Could you check a few things on this drawing? It's one solid part, dimensions in mm from its lowest x, y, z. Round coordinates to 2 decimals unless told otherwise and drop trailing zeros. Write each loop counter-clockwise with the first axis right and the second up, starting at its lowest first coordinate (ties: lowest second). Pieces come first, ordered by that corner, then holes. Notation, with made-up numbers: (45.25, 83.25) -> (68.25, 83.25) arc R27 cw to (68.25, 116.25) -> close; hole circle Ø2 at (72, -22.5). An arc over 180 degrees is marked (long way). Put each result on its own line as item: value. Start each with the question number.
1) I want a section at C-C, the plane y = 7.5. List the corners of the cut face in (x, z) for me (1 decimal).
2) I want a section at B-B, the plane x = 325. List the corners of the cut face in (y, z) for me (1 decimal).
3) I want a section at D-D, the plane z = 105. List the corners of the cut face in (x, y) for me, then the cut area to 3 significant figures.
4) Will these pins go through, and if not, where does the flat tip stop? P1, Ø3, axis at y = 6.5, z = 207.5, coming from the +X side (1 decimal); P2, Ø4, axis at x = 204.5, y = 5.5, coming from the +Z side; P3, Ø3, axis at x = 330, y = 4.5, coming from the -Z side.
5) If I drill on line 1 along X through (y, z) = (8.25, 291) (1 decimal); line 2 along Z through (x, y) = (43, 6.5); line 3 along X through (y, z) = (6.5, 330.5) (1 decimal), over which ranges is the centre line in solid material (lowest first)? Write a range as [from, to].
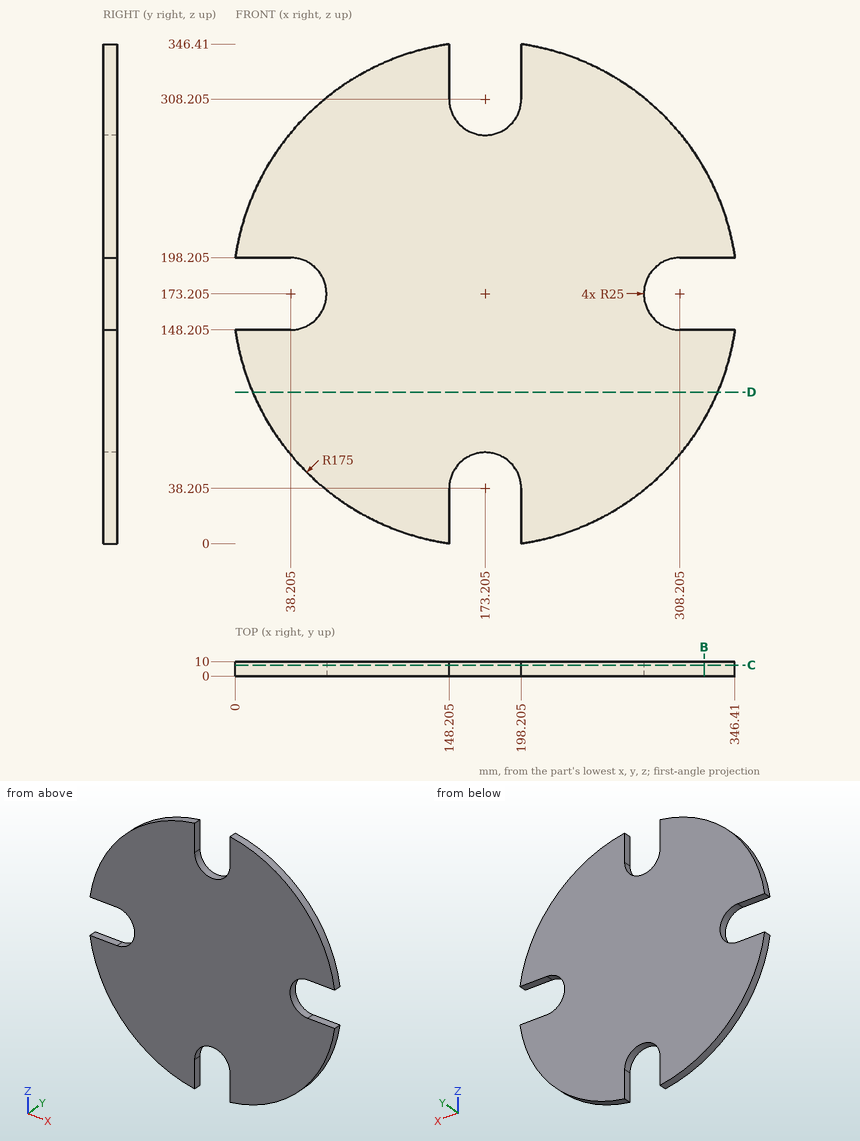
Findings:
1. outline: (0, 148.2) arc R175 ccw to (148.2, 0) -> (148.2, 38.2) arc R25 cw to (198.2, 38.2) -> (198.2, 0) arc R175 ccw to (346.4, 148.2) -> (308.2, 148.2) arc R25 cw to (308.2, 198.2) -> (346.4, 198.2) arc R175 ccw to (198.2, 346.4) -> (198.2, 308.2) arc R25 cw to (148.2, 308.2) -> (148.2, 346.4) arc R175 ccw to (0, 198.2) -> (38.2, 198.2) arc R25 cw to (38.2, 148.2) -> close
2. outline: (0, 86.1) -> (10, 86.1) -> (10, 148.2) -> (0, 148.2) -> close; (0, 198.2) -> (10, 198.2) -> (10, 260.3) -> (0, 260.3) -> close
3. outline: (12.04, 0) -> (334.37, 0) -> (334.37, 10) -> (12.04, 10) -> close
3. area: 3,220 mm2
4. P1: stops at x = 345.1
4. P2: stops at z = 345.74
4. P3: stops at z = 92.53
5. line 1: x = [43.8, 155.1], [191.3, 302.6]
5. line 2: z = [56.28, 148.67], [197.74, 290.13]
5. line 3: x = [96.5, 148.2], [198.2, 249.9]
